Design review of the part built by this model. Coordinates are the model's own, in mm. Face numbers are marked on the shaded views. A direction names the side the tool comes from. Give positions to 0.01 mm unless a question says otherwise; leave off trailing zeros. Loops run counter-clockwise (first coordinate to the right, second up) from the corner with the lowest first, then second, coordinate; pieces in that order, holes last.
from build123d import *

# Parameters (mm, degrees)
SKETCH1_W           = 24
SKETCH1_H           = 9
BOSS_EXTRUDE1_DEPTH = 30
FILLET1_R           = 1
FILLET2_R           = 3
SKETCH3_R           = 2.5
CUT_EXTRUDE2_DEPTH  = 10
SKETCH4_R           = 5
CUT_EXTRUDE3_DEPTH  = 4
SKETCH5_W           = 8
SKETCH5_H           = 5
BOSS_EXTRUDE2_DEPTH = 4
FILLET3_R           = 1


with BuildPart() as part:
    # Sketch1 → Boss-Extrude1 (new body)
    with BuildSketch(Plane.XY):
        Polygon((-18, -4.5), (-12, -4.5), (-12, 4.5), (-12, 14.5), (-18, 14.5), align=None)
        Rectangle(SKETCH1_W, SKETCH1_H)
        Polygon((12, 4.5), (12, -4.5), (18, -4.5), (18, 24.5), (12, 24.5), align=None)
    extrude(amount=BOSS_EXTRUDE1_DEPTH)

    # Fillet1
    fillet1_edges = [part.edges().sort_by_distance(p)[0] for p in [
        (-12, 4.5, 15),
        (12, 4.5, 15),
    ]]
    fillet(fillet1_edges, radius=FILLET1_R)

    # Fillet2
    fillet2_edges = [part.edges().sort_by_distance(p)[0] for p in [
        (18, 10, 0),
        (-18, 5, 0),
        (18, 10, 30),
        (-18, 5, 30),
    ]]
    fillet(fillet2_edges, radius=FILLET2_R)

    # Sketch3 → Cut-Extrude2 (cut)
    with BuildSketch(Plane(origin=(0, 4.5, 0), x_dir=(1, 0, 0), z_dir=(0, 1, 0))):
        with Locations(Location((0, -15, 0), (0, 0, 270))):
            Circle(SKETCH3_R)
    extrude(amount=-CUT_EXTRUDE2_DEPTH, mode=Mode.SUBTRACT)

    # Sketch4 → Cut-Extrude3 (cut)
    with BuildSketch(Plane(origin=(0, 4.5, 0), x_dir=(1, 0, 0), z_dir=(0, 1, 0))):
        with Locations(Location((0, -15, 0), (0, 0, 270))):
            Circle(SKETCH4_R)
    extrude(amount=-CUT_EXTRUDE3_DEPTH, mode=Mode.SUBTRACT)

    # Sketch5 → Boss-Extrude2 (add)
    with BuildSketch(Plane.XZ.offset(4.5)):
        with Locations((-14, 15)):
            Rectangle(SKETCH5_W, SKETCH5_H)
        with Locations((14, 15)):
            Rectangle(SKETCH5_W, SKETCH5_H)
    extrude(amount=BOSS_EXTRUDE2_DEPTH)

    # Fillet3
    fillet3_edges = [part.edges().sort_by_distance(p)[0] for p in [
        (14, -8.5, 17.5),
        (14, -8.5, 12.5),
        (-14, -8.5, 12.5),
        (-14, -8.5, 17.5),
    ]]
    fillet(fillet3_edges, radius=FILLET3_R)


solid = part.part
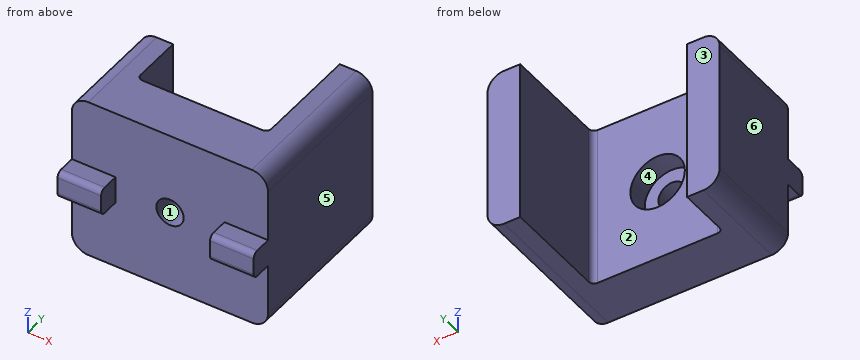
Q1. Take a section at D-D (y = 3.5). Give the boundary of the cut face in (x, z), plus the area to 3 significant figures.
Results:
outline: (-18, 3) arc R3 ccw to (-15, 0) - (15, 0) arc R3 ccw to (18, 3) - (18, 27) arc R3 ccw to (15, 30) - (-15, 30) arc R3 ccw to (-18, 27) - close; hole circle Ø10 at (0, 15)
area: 994 mm2
Q2. Take a section at C-C (z = 15). Give the boundary of the cut face in (x, y).
Results:
outline: (-18, -8.5) - (-10, -8.5) - (-10, -4.5) - (-2.5, -4.5) - (-2.5, 0.5) - (-5, 0.5) - (-5, 4.5) - (-11, 4.5) arc R1 cw to (-12, 5.5) - (-12, 14.5) - (-18, 14.5) - close; (2.5, -4.5) - (10, -4.5) - (10, -8.5) - (18, -8.5) - (18, 24.5) - (12, 24.5) - (12, 5.5) arc R1 cw to (11, 4.5) - (5, 4.5) - (5, 0.5) - (2.5, 0.5) - close
Q3. Tool access review of the marked faces 1, 2 and 3: name each direction out of +Z, -Z, +X, -X, +Y, -Y from which nothing blocks a thin tool from reaching the whole face with its end or side.
Results:
face 1: +Y, -Y
face 2: +Z, -Z, +Y
face 3: +Z, -Z, -X, +Y
Q4. Draft analysis for pull direction X (two halves, no side actions). For the marked faces 4, 5 and 6, state which applies: pulls with the +X half, pulls with the -X half, needs draft (parallel to the pull), parting line crosses it, or undercut.
Results:
face 4: undercut
face 5: pulls with the +X half
face 6: pulls with the -X half
Q5. Take a section at B-B (x = 0). Give the boundary of the cut face in (y, z), plus the area to 3 significant figures.
Results:
outline: (-4.5, 0) - (4.5, 0) - (4.5, 10) - (0.5, 10) - (0.5, 12.5) - (-4.5, 12.5) - close; (-4.5, 17.5) - (0.5, 17.5) - (0.5, 20) - (4.5, 20) - (4.5, 30) - (-4.5, 30) - close
area: 205 mm2
Q6. Insertion check: pin 1 (4 mm diameter, centred on x = -12.5, z = 12, fed in from +Y); pin 2 (6 mm diameter, centred on x = 0, z = 15, fed in from +Y); pin 3 (16 mm diameter, centred on x = 0, z = 15, fed in from +Y). Each pin has a flat end and moves straight along its axis. Give the tip position at first contact, or say it passes through.
Results:
pin 1: stops at y = 14.5
pin 2: stops at y = 0.5
pin 3: stops at y = 4.5
Q7. Take a section at A-A (y = 12.5). Give the boundary of the cut face in (x, z), plus the area to 3 significant figures.
Results:
outline: (-18, 3) arc R3 ccw to (-15, 0) - (-12, 0) - (-12, 30) - (-15, 30) arc R3 ccw to (-18, 27) - close; (12, 0) - (15, 0) arc R3 ccw to (18, 3) - (18, 27) arc R3 ccw to (15, 30) - (12, 30) - close
area: 352 mm2
Q8. Wall thickness on line 1 (X direction, y = -2, z = 15); line 2 (X direction, y = 9, z = 27); line 3 (Y direction, x = -8, z = 27.75): over which ranges is each line inside the solid? List them lowest first.
Results:
line 1: x = -18 to -2.5, 2.5 to 18
line 2: x = -18 to -12, 12 to 18
line 3: y = -4.5 to 4.5
